```python
from build123d import *

# Parameters (mm, degrees)
PAD_DEPTH            = 44.45
SKETCH002_R          = 35.052
POCKET_DEPTH         = 16.002
SKETCH003_R          = 4.826
PAD001_DEPTH         = 12.7
POLARPATTERN_COUNT   = 3
PAD002_DEPTH         = 9.525
SKETCH005_R          = 9.525
PAD003_DEPTH         = 12.7
SKETCH006_R          = 6.35
POCKET001_DEPTH      = 12.7
SKETCH007_W          = 95.705909
SKETCH007_H          = 12.7
PAD004_DEPTH         = 28.448
POCKET002_DEPTH      = 59.019352
POCKET002_DEPTH_BACK = -59.019352
SKETCH009_R          = 7.62
POCKET003_DEPTH      = 16.002


with BuildPart() as part:
    # Sketch → Pad (new body, symmetric)
    with BuildSketch(Plane.XZ):
        Polygon((38.1, -16.002), (123.698, -60.325), (139.7, -60.325), (139.7, 0), (38.1, 0), (0, 0), (0, -16.002), align=None)
    extrude(amount=PAD_DEPTH, both=True)

    # Sketch001 → Revolution (revolve)
    with BuildSketch(Plane.XZ):
        Polygon((44.45, 28.448), (44.45, -16.002), (34.798, -32.719754), (34.798, -60.452), (25.4, -60.452), (25.4, -32.719754), (35.052, -16.002), (35.052, 24.781826), (41.402, 28.448), align=None)
    revolve(axis=Axis((0, 0, 0), (0, 0, 1)))

    # Sketch002 → Pocket (cut)
    with BuildSketch(Plane.XY):
        Circle(SKETCH002_R)
    extrude(amount=-POCKET_DEPTH, mode=Mode.SUBTRACT)

    # Sketch003 (on DatumPlane) → Pad001 (join)
    with BuildSketch(Plane.XY.offset(25.4)):
        with BuildLine():
            ThreePointArc((-59.059347, 9.331667), (-66.675, 1.8e-05), (-59.059383, -9.33166))
            Line((-42.597095, -12.7), (-59.059383, -9.33166))
            Line((-42.597095, 12.7), (-42.597095, -12.7))
            Line((-59.059347, 9.331667), (-42.597095, 12.7))
        make_face()
        with Locations((-57.15, 0)):
            Circle(SKETCH003_R, mode=Mode.SUBTRACT)
    pad001 = extrude(amount=-PAD001_DEPTH)

    # PolarPattern: Pad001 ×3 about axis
    polarpattern_axis = Axis((0, 0, 25.4), (0, 0, 1))
    for i in range(1, POLARPATTERN_COUNT):
        add(pad001.rotate(polarpattern_axis, i * 360 / POLARPATTERN_COUNT))

    # Sketch004 (on DatumPlane) → Pad002 (join, symmetric)
    with BuildSketch(Plane.XY.offset(0.125)):
        Polygon((-35.052, 3.175), (-3.175, 3.175), (-3.175, 35.052), (3.175, 35.052), (3.175, 3.175), (35.052, 3.175), (35.052, -3.175), (3.175, -3.175), (3.175, -35.052), (-3.175, -35.052), (-3.175, -3.175), (-35.052, -3.175), align=None)
    extrude(amount=PAD002_DEPTH, both=True)

    # Sketch005 (on DatumPlane) → Pad003 (join, symmetric)
    with BuildSketch(Plane.XY.offset(0.125)):
        Circle(SKETCH005_R)
    extrude(amount=PAD003_DEPTH, both=True)

    # Sketch006 (on DatumPlane) → Pocket001 (cut, symmetric)
    with BuildSketch(Plane.XY.offset(0.125)):
        Circle(SKETCH006_R)
    extrude(amount=POCKET001_DEPTH, both=True, mode=Mode.SUBTRACT)

    # Sketch007 → Pad004 (join)
    with BuildSketch(Plane.XY):
        with Locations((91.847045, 0)):
            Rectangle(SKETCH007_W, SKETCH007_H)
    extrude(amount=PAD004_DEPTH)

    # Sketch008 → Pocket002 (cut, two sides)
    with BuildSketch(Plane.XZ) as pocket002_sk:
        Polygon((44.45, 28.448), (139.7, 0), (139.7, 28.448), align=None)
    extrude(amount=-POCKET002_DEPTH, mode=Mode.SUBTRACT)
    extrude(pocket002_sk.sketch, amount=-POCKET002_DEPTH_BACK, mode=Mode.SUBTRACT)

    # Sketch009 (on DatumPlane) → Pocket003 (cut)
    with BuildSketch(Plane.YZ.offset(139.7)):
        with Locations((-19.05, -32.766)):
            Circle(SKETCH009_R)
        with Locations((19.05, -32.766)):
            Circle(SKETCH009_R)
    extrude(amount=-POCKET003_DEPTH, mode=Mode.SUBTRACT)


solid = part.part
```
Geometry: final body of the model. Coordinates: model frame, mm. A direction names the side the tool comes from. Round coordinates to 2 decimals unless told otherwise and drop trailing zeros. Order: outer loops, then holes, each group sorted by start corner. A loop starts at its lowest first (then second) coordinate and runs counter-clockwise, first axis right, second up. Notation, with made-up numbers: M 71,77 L 111,77 A17 cw 111,85 Z; hole C -26.5,21 d1. An arc over 180 degrees is marked long. One line per item, written item: value.
(1) Line query: probe 1 along Y at (x, z) = (1, 21); probe 2 along X at (y, z) = (-4, -21.5); probe 3 along X at (y, z) = (-5, -35). Output: solid intervals per line, ascending. Write a range as [from, to].
Result sheet:
probe 1: [-44.44, -35.04], [35.04, 44.44]
probe 2: [-41.08, -31.63], [31.63, 41.08], [48.72, 139.7]
probe 3: [-34.44, -24.9], [24.9, 34.44], [74.79, 139.7]
(2) Cut plane D-D (y = -17.5). Give the number of separate pieces and of enclosed holes in the cut face, and give its area (3 significant figures).
Result sheet:
separate pieces: 3
enclosed holes: 0
area: 5,990 mm2
(3) Cut plane C-C (x = 114.5). Return the cut outline in (y, z), and give its area (3 significant figures).
Result sheet:
outline: M -44.45,-55.56 L 44.45,-55.56 L 44.45,0 L 6.35,0 L 6.35,7.53 L -6.35,7.53 L -6.35,0 L -44.45,0 Z
area: 5,040 mm2
(4) Pin query (flat end, axial travel): P1, Ø6, axis at y = 16.5, z = 8, coming from the -X side; P2, Ø5.5, axis at x = 19, z = -2, coming from the +Y side; P3, Ø4, axis at y = 19.5, z = 13.5, coming from the -X side. Return the tip coordinate at first contact, or that it passes through.
Result sheet:
P1: x = -42.35
P2: y = 44.45
P3: x = -40.86
(5) Cut plane A-A (z = 18). Return the cut outline in (x, y) (3 decimals), and give its area (3 significant figures).
Result sheet:
outline: M -59.059,-9.332 L -42.597,-12.7 A44.45 ccw 10.3,-43.24 L 21.448,-55.813 A9.525 ccw 37.611,-46.481 L 32.297,-30.54 A44.45 ccw 43.994,-6.35 L 79.432,-6.35 L 79.432,6.35 L 43.994,6.35 A44.45 ccw 32.297,30.54 L 37.611,46.481 A9.525 ccw 21.448,55.813 L 10.3,43.24 A44.45 ccw -42.597,12.7 L -59.059,9.332 A9.525 ccw Z; hole C -57.15,0 d9.652; hole C 0,0 d70.104; hole C 28.575,-49.493 d9.652; hole C 28.575,49.493 d9.652
area: 3,890 mm2
(6) Cut plane B-B (z = -43). Return the cut outline in (x, y).
Result sheet:
outline: C 0,0 d69.6; M 90.24,-44.45 L 139.7,-44.45 L 139.7,44.45 L 90.24,44.45 Z; hole C 0,0 d50.8
(7) Pull-direction query (Y, two-part tool) for faces 5 (the flat face through (81, -6.35, 11)), 6 (the flat face through (26, 45, 25.4)), 7 (the cylindrical face through (-61.97, 0.21, 19.14)); classes: pulls with the +Y half, pulls with the -Y half, needs draft (parallel to the pull), parting line crosses it, or undercut.
Result sheet:
face 5: pulls with the -Y half
face 6: needs draft
face 7: undercut
(8) Reachability of faces 1 (the flat face through (29, -39, -16.002)), 2 (the cylindrical face through (131.81, -11.78, -30.48)), 3 (the flat face through (2, -6.2, -12.575)), 4 (the flat face through (0, -22, 9.65)) from +Z, -Z, +X, -X, +Y, -Y: full face, straight path, thin tool, end or side. Return the list, or none.
Result sheet:
face 1: -Z, -Y
face 2: +X
face 3: -Z
face 4: +Z
